The listing builds one solid part. Answer for the finished solid, in the listing's coordinates (mm). A direction names the side the tool comes from. Give positions to 0.01 mm unless a question says otherwise; leave off trailing zeros. Loops run counter-clockwise (first coordinate to the right, second up) from the corner with the lowest first, then second, coordinate; pieces in that order, holes last. Notation, with made-up numbers: (-39, 27) - (-6, 27) arc R17 cw to (-6, 41) - close; hole circle Ø10 at (23.25, -4). An arc over 180 degrees is marked (long way). One line per item, written item: value. Start each with the question number.
from build123d import *

# Parameters (mm, degrees)
CUT_EXTRUDE_1_DEPTH = 64
CUT_EXTRUDE_START   = -64
CUT_EXTRUDE_2_DEPTH = 64
SKETCH_4_W          = 74
SKETCH_4_H          = 76
EXTRUDE_1_DEPTH     = 10
EXTRUDE_START       = -66
SKETCH_5_R          = 5
EXTRUDE_2_DEPTH     = 10
SKETCH_5_3_R        = 5
EXTRUDE_3_DEPTH     = 10


with BuildPart() as part:
    # Sketch 1 → Revolve 1 (revolve)
    with BuildSketch(Plane(origin=(0, 0, 0), x_dir=(1, 0, 0), z_dir=(0, 1, 0))):
        Polygon((74.878584377, 0), (-70.121415623, 0), (-70.121415623, -30), (-59.121415623, -30), (-59.121415623, -21), (-30.121415623, -21), (-30.121415623, -17.5), (74.878584377, -17.5), align=None)
    revolve(axis=Axis((-70.121415623, 0, 0), (1, 0, 0)))

    # Sketch 2 → Cut-Extrude 1 (cut)
    with BuildSketch(Plane(origin=(74.878584377, 0, 0), x_dir=(0, 0, -1), z_dir=(1, 0, 0))):
        with BuildLine():
            Line((-15.811388301, 7.5), (15.811388301, 7.5))
            ThreePointArc((15.811388301, 7.5), (0, 17.5), (-15.811388301, 7.5))
        make_face()
    extrude(amount=-CUT_EXTRUDE_1_DEPTH, mode=Mode.SUBTRACT)

    # Sketch 3 → Cut-Extrude 2 (cut)
    with BuildSketch(Plane.ZY.offset(70.121415623).offset(CUT_EXTRUDE_START)):
        with BuildLine():
            Line((14.966629547, -26), (-14.966629547, -26))
            ThreePointArc((-14.966629547, -26), (0, -30), (14.966629547, -26))
        make_face()
        with BuildLine():
            ThreePointArc((14.966629547, 26), (0, 30), (-14.966629547, 26))
            Line((-14.966629547, 26), (14.966629547, 26))
        make_face()
    extrude(amount=CUT_EXTRUDE_2_DEPTH, mode=Mode.SUBTRACT)

    # Sketch 4 → Extrude 1 (add)
    # profile 1 of 2: a face of its own
    with BuildSketch(Plane.ZY.offset(70.121415623)):
        Rectangle(SKETCH_4_W, SKETCH_4_H)
        with BuildLine():
            ThreePointArc((-14.966629547, 26), (-30, 0), (-14.966629547, -26))
            Line((-14.966629547, -26), (14.966629547, -26))
            ThreePointArc((14.966629547, -26), (30, 0), (14.966629547, 26))
            Line((14.966629547, 26), (-14.966629547, 26))
        make_face(mode=Mode.SUBTRACT)
    # profile 2 of 2: a face of its own
    with BuildSketch(Plane.ZY.offset(70.121415623)):
        with BuildLine():
            Line((14.966629547, 26), (-14.966629547, 26))
            ThreePointArc((-14.966629547, 26), (-30, 0), (-14.966629547, -26))
            Line((-14.966629547, -26), (14.966629547, -26))
            ThreePointArc((14.966629547, -26), (30, 0), (14.966629547, 26))
        make_face()
    extrude(amount=EXTRUDE_1_DEPTH)

    # Sketch 5 → Extrude 2 (add)
    with BuildSketch(Plane(origin=(0, 38, 0), x_dir=(1, 0, 0), z_dir=(0, 1, 0)).offset(EXTRUDE_START)):
        with BuildLine():
            Line((-80.121415623, 37), (-129.550289518, 13.552475067))
            ThreePointArc((-129.550289518, 13.552475067), (-138.120501498, -0.165598609), (-129.249504521, -13.691111221))
            Line((-129.249504521, -13.691111221), (-80.121415623, -37))
            Line((-80.121415623, -37), (-80.121415623, 37))
        make_face()
        with Locations(Location((-123.121415623, 0, 0), (0, 0, 270))):
            Circle(SKETCH_5_R, mode=Mode.SUBTRACT)
    extrude(amount=-EXTRUDE_2_DEPTH)

    # Sketch 5_3 → Extrude 3 (add)
    with BuildSketch(Plane(origin=(0, 38, 0), x_dir=(1, 0, 0), z_dir=(0, 1, 0))):
        with BuildLine():
            Line((-80.121415623, 37), (-129.550289518, 13.552475067))
            ThreePointArc((-129.550289518, 13.552475067), (-138.120501498, -0.165598609), (-129.249504521, -13.691111221))
            Line((-129.249504521, -13.691111221), (-80.121415623, -37))
            Line((-80.121415623, -37), (-80.121415623, 37))
        make_face()
        with Locations(Location((-123.121415623, 0, 0), (0, 0, 270))):
            Circle(SKETCH_5_3_R, mode=Mode.SUBTRACT)
    extrude(amount=-EXTRUDE_3_DEPTH)


solid = part.part
1. A cutting plane is placed at C-C (y = 0). Determine the outline of the cut face in (x, z).
2. For faces 1 (the cylindrical face through (-44.42, -6.31, 20.03)), 2 (the flat face through (-103, -28, -1)), 3 (the cylindrical face through (-65, 0, 30)), 4 (the flat face through (10.879, 11, 0)), determine the directions among +Z, -Z, +X, -X, +Y, -Y from which every point of the face is accessible in a straight line to the end or side of a thin tool.
3. A cutting plane is placed at D-D (x = -27.5). Determine the outline of the cut face in (y, z), plus the area to 3 significant figures.
4. A cutting plane is placed at B-B (y = 31). Determine the outline of the cut face in (x, z), plus the area to 3 significant figures.
5. A cutting plane is placed at A-A (z = 0). Give the number of separate pieces and of enclosed holes in the cut face, plus the area to 4 significant figures.
6. Find the intervals of material crossed by L1, parallel to X at y = -34.75, z = 0; L2, parallel to Y at x = -93, z = 0.5; L3, parallel to X at y = -19.5, z = -32.5, in increasing order. Write a range as [from, to].
7. Determine the mould class of faces 5 (the cylindrical face through (-127.557, 33.07, 2.307)), 6 (the flat face through (-97, -38, -1)), 7 (the flat face through (-105.03, -32.93, 25.18)) for opening direction X: released by +X, released by -X, zero draft, split by the parting line, or undercut.
8. Flat-ended cylindrical pins translate along their axes: pin 1 (8 mm diameter, centred on y = 13, z = -2.5, fed in from +X); pin 2 (5.5 mm diameter, centred on x = -66.5, z = 4.5, fed in from -Y); pin 3 (2 mm diameter, centred on y = -19, z = 27, fed in from -X). Find the tip coordinate at first contact, or state that the pin passes through.
Results below:
1. outline: (-80.12, -37) - (-70.12, -37) - (-70.12, -30) - (-59.12, -30) - (-59.12, -21) - (-30.12, -21) - (-30.12, -17.5) - (74.88, -17.5) - (74.88, 17.5) - (-30.12, 17.5) - (-30.12, 21) - (-59.12, 21) - (-59.12, 30) - (-70.12, 30) - (-70.12, 37) - (-80.12, 37) - close
2. face 1: +X
2. face 2: +Z, -Z, -X
2. face 3: +Z, +X
2. face 4: +Z, -Z, +X, +Y
3. outline: circle Ø35 at (0, 0)
3. area: 962 mm^2
4. outline: (-129.55, -13.55) - (-80.12, -37) - (-70.12, -37) - (-70.12, 37) - (-80.12, 37) - (-129.25, 13.69) arc R15 ccw to start; hole circle Ø10 at (-123.12, 0)
4. area: 3,330 mm^2
5. separate pieces: 3
5. enclosed holes: 0
5. area: 6,545 mm^2
6. L1: x = [-138.12, -128.12], [-118.12, -70.12]
6. L2: y = [-38, -28], [28, 38]
6. L3: x = [-80.12, -70.12]
7. face 5: undercut
7. face 6: zero draft
7. face 7: released by -X
8. pin 1: stops at x = 10.88
8. pin 2: stops at y = -26
8. pin 3: stops at x = -80.12
